Geometry: final body of the model. Coordinates: model frame, mm. Coordinates: 2 decimals unless noted, no trailing zeros. Order: outer loops, then holes, each group sorted by start corner. A loop starts at its lowest first (then second) coordinate and runs counter-clockwise, first axis right, second up. Notation, with made-up numbers: (66.25, -22) -> (88.25, -22) arc R18 ccw to (88.25, -13) -> close; hole circle Ø2 at (31.25, 19). An arc over 180 degrees is marked (long way). Answer in a Markdown table with one row per item. Add a question column.
1) Section query B-B on z = 29. Return the cut outline in (x, y) (3 decimals), then the cut area to 3 significant figures.
2) Section query C-C on x = 15.55. Return the cut outline in (y, z) (3 decimals).
3) Contact query for a flat-ended pin moving along its axis: P1, Ø3, axis at x = -3, z = -8.5, coming from the -Y side. Output: stop coordinate, or through.
4) Ray query, line 1 (X direction, y = 0.85, z = 29) (3 decimals); line 2 (Z direction, x = -7.45, y = 1.25) (3 decimals); line 3 (Z direction, x = -14.5, y = 0.7). Return the intervals inside material, ascending. Write a range as from..to.
5) Section query A-A on x = -7.45. Return the cut outline in (y, z) (3 decimals).
6) Pull-direction query (X, two-part tool) for faces 1 (the face through (15.67, 0.84, 46.05)), 2 (the face through (19.05, 1, 1)), 3 (the face through (-19.05, 1, -1)), 4 (the face through (0, 0, 1)); classes: +X half, -X half, draft (parallel to the pull), parting line (faces both ways), or undercut.
Autodesk Inventor part; units mm, degrees
ref_plane "YZ Plane" through (0, 0, 0) normal (1, 0, 0) x (0, 1, 0)
ref_plane "XZ Plane" through (0, 0, 0) normal (0, 1, 0) x (-1, 0, 0)
ref_plane "XY Plane" through (0, 0, 0) normal (0, 0, 1) x (1, 0, 0)
sketch "Sketch1" plane through (0, 0, 0) normal (0, 1, 0) x (-1, 0, 0)
  line L0 (19.05, 50.8) -> (6.35, 50.8)
  line L1 (6.35, -50.8) -> (19.05, -50.8)
  line L2 (19.05, -50.8) -> (19.05, 50.8)
  line L3 (6.35, 50.8) -> (-19.05, 50.8)
  line L4 (-19.05, 50.8) -> (-19.05, -50.8)
  line L5 (-19.05, -50.8) -> (6.35, -50.8)
  line L6 (6.35, -50.8) -> (6.35, -50.8)
  line L7 (6.35, 50.8) -> (6.35, 50.8)
  point P0 (0, 0)
  dimension "d0" = 101.6
  dimension "d2" = 101.6
  dimension "d3" = 0
  dimension "d4" = 12.7
  dimension "d5" = 25.4
  dimension "d6" = 0
  dimension "d7" = 50.8
  dimension "d8" = 38.1
  dimension "d9" = 19.05
  dimension "d10" = 12.7
extrude "Extrusion1" add sketch "Sketch1" along normal blind 1.651
sketch "Sketch2" plane through (0, 1.651, 0) normal (0, 1, 0) x (1, 0, 0)
  circle A0 centre (-15.875, -47.625) radius 1.5875
  circle A1 centre (15.875, -47.625) radius 1.5875
  circle A2 centre (-15.875, 47.625) radius 1.5875
  circle A3 centre (15.875, 47.625) radius 1.5875
  line L0 (19.05, 50.8) -> (-19.05, 50.8)
  line L1 (-19.05, 50.8) -> (-19.05, -50.8)
  line L2 (19.05, -50.8) -> (19.05, 50.8)
  line L3 (-19.05, -50.8) -> (19.05, -50.8)
  point P0 (0, 0)
  point P1 (-6.35, 38.1)
  dimension "d13" = 3.175
  dimension "d14" = 3.175
  dimension "d15" = 3.175
  dimension "d16" = 3.175
  dimension "d17" = 3.175
  dimension "d18" = 3.175
  dimension "d19" = 3.175
  dimension "d20" = 3.175
  dimension "d21" = 3.175
  dimension "d22" = 3.175
  dimension "d23" = 3.175
  dimension "d27" = 3.175
extrude "Extrusion2" cut sketch "Sketch2" against normal through all contours A0 | A1 | A2 | A3
sketch "Sketch3" plane through (0, 1.651, 0) normal (0, 1, 0) x (1, 0, 0)
  circle A0 centre (-7.45, 29) radius 1.375
  circle A1 centre (15.55, 29) radius 1.375
  circle A2 centre (-7.45, -29) radius 1.375
  circle A3 centre (15.55, -29) radius 1.375
  line L0 (-19.05, -50.8) -> (19.05, -50.8)
  line L1 (19.05, 50.8) -> (-19.05, 50.8)
  line L2 (-19.05, 50.8) -> (-19.05, -50.8)
  line L3 (19.05, -50.8) -> (19.05, 50.8)
  point P0 (0, 0)
  dimension "d28" = 2.75
  dimension "d29" = 2.75
  dimension "d30" = 2.75
  dimension "d31" = 2.75
  dimension "d32" = 23
  dimension "d33" = 23
  dimension "d34" = 58
  dimension "d35" = 101.6
  dimension "d36" = 29
  dimension "d39" = 0
  dimension "d40" = 0
  dimension "d41" = 58
  dimension "d44" = 3.5
extrude "Extrusion3" cut sketch "Sketch3" against normal through all contours A0 | A1 | A2 | A3
equation "\"d0\" = d2"
equation "\"d6\" = d3"
equation "\"d10\" = d4"
equation "\"d14\" = d13"
equation "\"d15\" = d13"
equation "\"d16\" = d13"
equation "\"d19\" = d18"
equation "\"d20\" = d17"
equation "\"d21\" = d19"
equation "\"d22\" = d17"
equation "\"d23\" = d17"
equation "\"d27\" = d21"
equation "\"d29\" = d28"
equation "\"d30\" = d28"
equation "\"d31\" = d28"
equation "\"d32\" = d33"
equation "\"d41\" = d34"
properties part number "STARduino layout"
Result:
| question | item | result |
|---|---|---|
| 1 | outline | (-19.05, 0) -> (-8.825, 0) -> (-8.825, 1.651) -> (-19.05, 1.651) -> close; (-6.075, 0) -> (14.175, 0) -> (14.175, 1.651) -> (-6.075, 1.651) -> close; (16.925, 0) -> (19.05, 0) -> (19.05, 1.651) -> (16.925, 1.651) -> close |
| 1 | area | 53.8 mm2 |
| 2 | outline | (0, -50.8) -> (1.651, -50.8) -> (1.651, -49.179) -> (0, -49.179) -> close; (0, -46.071) -> (1.651, -46.071) -> (1.651, -30.375) -> (0, -30.375) -> close; (0, -27.625) -> (1.651, -27.625) -> (1.651, 27.625) -> (0, 27.625) -> close; (0, 30.375) -> (1.651, 30.375) -> (1.651, 46.071) -> (0, 46.071) -> close; (0, 49.179) -> (1.651, 49.179) -> (1.651, 50.8) -> (0, 50.8) -> close |
| 3 | P1 | y = 0 |
| 4 | line 1 | -19.05..-8.825, -6.075..14.175, 16.925..19.05 |
| 4 | line 2 | -50.8..-30.375, -27.625..27.625, 30.375..50.8 |
| 4 | line 3 | -50.8..-48.42, -46.83..46.83, 48.42..50.8 |
| 5 | outline | (0, -50.8) -> (1.651, -50.8) -> (1.651, -30.375) -> (0, -30.375) -> close; (0, -27.625) -> (1.651, -27.625) -> (1.651, 27.625) -> (0, 27.625) -> close; (0, 30.375) -> (1.651, 30.375) -> (1.651, 50.8) -> (0, 50.8) -> close |
| 6 | face 1 | undercut |
| 6 | face 2 | +X half |
| 6 | face 3 | -X half |
| 6 | face 4 | draft |
